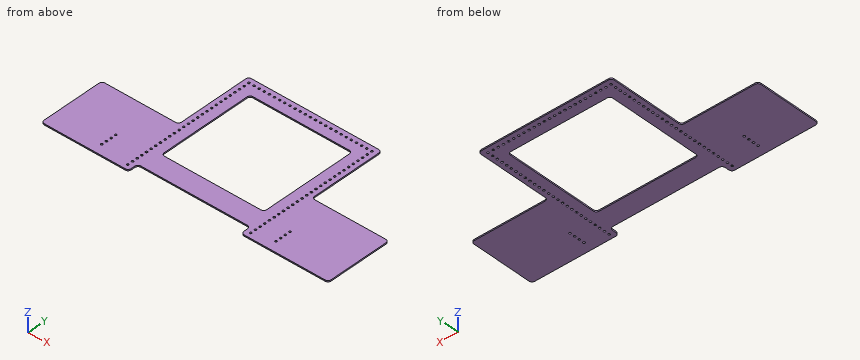
```python
from build123d import *

# Parameters (mm, degrees)
SKETCH1_R           = 2.54
SKETCH1_W           = 254
SKETCH1_H           = 241.3
BOSS_EXTRUDE1_DEPTH = 3.175
FILLET1_R           = 7.62


with BuildPart() as part:
    # Sketch1 → Boss-Extrude1 (new body)
    with BuildSketch(Plane.XY):
        Polygon((392.015739824, -380.530659381), (607.915739824, -380.530659381), (607.915739824, -215.553323478), (417.415739824, -215.553323478), (417.415739824, -25.053323478), (87.215739824, -25.053323478), (87.215739824, -215.553323478), (-103.284260176, -215.553323478), (-103.284260176, -380.530659381), (112.615739824, -380.530659381), (112.615739824, -355.253323478), (392.015739824, -355.253323478), align=None)
        with Locations((99.915739824, -37.753323478)):
            Circle(SKETCH1_R, mode=Mode.SUBTRACT)
        with Locations((112.615739824, -37.753323478)):
            Circle(SKETCH1_R, mode=Mode.SUBTRACT)
        with Locations((125.315739824, -37.753323478)):
            Circle(SKETCH1_R, mode=Mode.SUBTRACT)
        with Locations((138.015739824, -37.753323478)):
            Circle(SKETCH1_R, mode=Mode.SUBTRACT)
        with Locations((150.715739824, -37.753323478)):
            Circle(SKETCH1_R, mode=Mode.SUBTRACT)
        with Locations((163.415739824, -37.753323478)):
            Circle(SKETCH1_R, mode=Mode.SUBTRACT)
        with Locations((176.115739824, -37.753323478)):
            Circle(SKETCH1_R, mode=Mode.SUBTRACT)
        with Locations((188.815739824, -37.753323478)):
            Circle(SKETCH1_R, mode=Mode.SUBTRACT)
        with Locations((201.515739824, -37.753323478)):
            Circle(SKETCH1_R, mode=Mode.SUBTRACT)
        with Locations((214.215739824, -37.753323478)):
            Circle(SKETCH1_R, mode=Mode.SUBTRACT)
        with Locations((226.915739824, -37.753323478)):
            Circle(SKETCH1_R, mode=Mode.SUBTRACT)
        with Locations((239.615739824, -37.753323478)):
            Circle(SKETCH1_R, mode=Mode.SUBTRACT)
        with Locations((252.315739824, -37.753323478)):
            Circle(SKETCH1_R, mode=Mode.SUBTRACT)
        with Locations((265.015739824, -37.753323478)):
            Circle(SKETCH1_R, mode=Mode.SUBTRACT)
        with Locations((277.715739824, -37.753323478)):
            Circle(SKETCH1_R, mode=Mode.SUBTRACT)
        with Locations((290.415739824, -37.753323478)):
            Circle(SKETCH1_R, mode=Mode.SUBTRACT)
        with Locations((303.115739824, -37.753323478)):
            Circle(SKETCH1_R, mode=Mode.SUBTRACT)
        with Locations((315.815739824, -37.753323478)):
            Circle(SKETCH1_R, mode=Mode.SUBTRACT)
        with Locations((328.515739824, -37.753323478)):
            Circle(SKETCH1_R, mode=Mode.SUBTRACT)
        with Locations((341.215739824, -37.753323478)):
            Circle(SKETCH1_R, mode=Mode.SUBTRACT)
        with Locations((353.915739824, -37.753323478)):
            Circle(SKETCH1_R, mode=Mode.SUBTRACT)
        with Locations((366.615739824, -37.753323478)):
            Circle(SKETCH1_R, mode=Mode.SUBTRACT)
        with Locations((379.315739824, -37.753323478)):
            Circle(SKETCH1_R, mode=Mode.SUBTRACT)
        with Locations((392.015739824, -37.753323478)):
            Circle(SKETCH1_R, mode=Mode.SUBTRACT)
        with Locations((404.715739824, -37.753323478)):
            Circle(SKETCH1_R, mode=Mode.SUBTRACT)
        with Locations((99.915739824, -50.453323478)):
            Circle(SKETCH1_R, mode=Mode.SUBTRACT)
        with Locations((99.915739824, -63.153323478)):
            Circle(SKETCH1_R, mode=Mode.SUBTRACT)
        with Locations((99.915739824, -75.853323478)):
            Circle(SKETCH1_R, mode=Mode.SUBTRACT)
        with Locations((99.915739824, -88.553323478)):
            Circle(SKETCH1_R, mode=Mode.SUBTRACT)
        with Locations((99.915739824, -101.253323478)):
            Circle(SKETCH1_R, mode=Mode.SUBTRACT)
        with Locations((99.915739824, -113.953323478)):
            Circle(SKETCH1_R, mode=Mode.SUBTRACT)
        with Locations((99.915739824, -126.653323478)):
            Circle(SKETCH1_R, mode=Mode.SUBTRACT)
        with Locations((99.915739824, -139.353323478)):
            Circle(SKETCH1_R, mode=Mode.SUBTRACT)
        with Locations((99.915739824, -152.053323478)):
            Circle(SKETCH1_R, mode=Mode.SUBTRACT)
        with Locations((99.915739824, -164.753323478)):
            Circle(SKETCH1_R, mode=Mode.SUBTRACT)
        with Locations((99.915739824, -177.453323478)):
            Circle(SKETCH1_R, mode=Mode.SUBTRACT)
        with Locations((99.915739824, -190.153323478)):
            Circle(SKETCH1_R, mode=Mode.SUBTRACT)
        with Locations((99.915739824, -202.853323478)):
            Circle(SKETCH1_R, mode=Mode.SUBTRACT)
        with Locations((99.915739824, -215.553323478)):
            Circle(SKETCH1_R, mode=Mode.SUBTRACT)
        with Locations((99.915739824, -228.253323478)):
            Circle(SKETCH1_R, mode=Mode.SUBTRACT)
        with Locations((99.915739824, -240.953323478)):
            Circle(SKETCH1_R, mode=Mode.SUBTRACT)
        with Locations((99.915739824, -253.653323478)):
            Circle(SKETCH1_R, mode=Mode.SUBTRACT)
        with Locations((99.915739824, -266.353323478)):
            Circle(SKETCH1_R, mode=Mode.SUBTRACT)
        with Locations((99.915739824, -279.053323478)):
            Circle(SKETCH1_R, mode=Mode.SUBTRACT)
        with Locations((99.915739824, -291.753323478)):
            Circle(SKETCH1_R, mode=Mode.SUBTRACT)
        with Locations((99.915739824, -304.453323478)):
            Circle(SKETCH1_R, mode=Mode.SUBTRACT)
        with Locations((99.915739824, -317.153323478)):
            Circle(SKETCH1_R, mode=Mode.SUBTRACT)
        with Locations((99.915739824, -329.853323478)):
            Circle(SKETCH1_R, mode=Mode.SUBTRACT)
        with Locations((99.915739824, -342.553323478)):
            Circle(SKETCH1_R, mode=Mode.SUBTRACT)
        with Locations((99.915739824, -355.253323478)):
            Circle(SKETCH1_R, mode=Mode.SUBTRACT)
        with Locations((99.915739824, -367.953323478)):
            Circle(SKETCH1_R, mode=Mode.SUBTRACT)
        with Locations((404.715739824, -50.453323478)):
            Circle(SKETCH1_R, mode=Mode.SUBTRACT)
        with Locations((404.715739824, -63.153323478)):
            Circle(SKETCH1_R, mode=Mode.SUBTRACT)
        with Locations((404.715739824, -75.853323478)):
            Circle(SKETCH1_R, mode=Mode.SUBTRACT)
        with Locations((404.715739824, -88.553323478)):
            Circle(SKETCH1_R, mode=Mode.SUBTRACT)
        with Locations((404.715739824, -101.253323478)):
            Circle(SKETCH1_R, mode=Mode.SUBTRACT)
        with Locations((404.715739824, -113.953323478)):
            Circle(SKETCH1_R, mode=Mode.SUBTRACT)
        with Locations((404.715739824, -126.653323478)):
            Circle(SKETCH1_R, mode=Mode.SUBTRACT)
        with Locations((404.715739824, -139.353323478)):
            Circle(SKETCH1_R, mode=Mode.SUBTRACT)
        with Locations((404.715739824, -152.053323478)):
            Circle(SKETCH1_R, mode=Mode.SUBTRACT)
        with Locations((404.715739824, -164.753323478)):
            Circle(SKETCH1_R, mode=Mode.SUBTRACT)
        with Locations((404.715739824, -177.453323478)):
            Circle(SKETCH1_R, mode=Mode.SUBTRACT)
        with Locations((404.715739824, -190.153323478)):
            Circle(SKETCH1_R, mode=Mode.SUBTRACT)
        with Locations((404.715739824, -202.853323478)):
            Circle(SKETCH1_R, mode=Mode.SUBTRACT)
        with Locations((404.715739824, -215.553323478)):
            Circle(SKETCH1_R, mode=Mode.SUBTRACT)
        with Locations((404.715739824, -228.253323478)):
            Circle(SKETCH1_R, mode=Mode.SUBTRACT)
        with Locations((404.715739824, -240.953323478)):
            Circle(SKETCH1_R, mode=Mode.SUBTRACT)
        with Locations((404.715739824, -253.653323478)):
            Circle(SKETCH1_R, mode=Mode.SUBTRACT)
        with Locations((404.715739824, -266.353323478)):
            Circle(SKETCH1_R, mode=Mode.SUBTRACT)
        with Locations((404.715739824, -279.053323478)):
            Circle(SKETCH1_R, mode=Mode.SUBTRACT)
        with Locations((404.715739824, -291.753323478)):
            Circle(SKETCH1_R, mode=Mode.SUBTRACT)
        with Locations((404.715739824, -304.453323478)):
            Circle(SKETCH1_R, mode=Mode.SUBTRACT)
        with Locations((404.715739824, -317.153323478)):
            Circle(SKETCH1_R, mode=Mode.SUBTRACT)
        with Locations((404.715739824, -329.853323478)):
            Circle(SKETCH1_R, mode=Mode.SUBTRACT)
        with Locations((404.715739824, -342.553323478)):
            Circle(SKETCH1_R, mode=Mode.SUBTRACT)
        with Locations((404.715739824, -355.253323478)):
            Circle(SKETCH1_R, mode=Mode.SUBTRACT)
        with Locations((404.715739824, -367.953323478)):
            Circle(SKETCH1_R, mode=Mode.SUBTRACT)
        with Locations((23.715739824, -317.153323478)):
            Circle(SKETCH1_R, mode=Mode.SUBTRACT)
        with Locations((455.515739824, -317.153323478)):
            Circle(SKETCH1_R, mode=Mode.SUBTRACT)
        with Locations((455.515739824, -329.853323478)):
            Circle(SKETCH1_R, mode=Mode.SUBTRACT)
        with Locations((455.515739824, -342.553323478)):
            Circle(SKETCH1_R, mode=Mode.SUBTRACT)
        with Locations((455.515739824, -355.253323478)):
            Circle(SKETCH1_R, mode=Mode.SUBTRACT)
        with Locations((23.715739824, -329.853323478)):
            Circle(SKETCH1_R, mode=Mode.SUBTRACT)
        with Locations((23.715739824, -342.553323478)):
            Circle(SKETCH1_R, mode=Mode.SUBTRACT)
        with Locations((23.715739824, -355.253323478)):
            Circle(SKETCH1_R, mode=Mode.SUBTRACT)
        with Locations((252.315739824, -183.803323478)):
            Rectangle(SKETCH1_W, SKETCH1_H, mode=Mode.SUBTRACT)
    extrude(amount=BOSS_EXTRUDE1_DEPTH)

    # Fillet1
    fillet1_edges = [part.edges().sort_by_distance(p)[0] for p in [
        (607.915739824, -380.530659381, 1.5875),
        (392.015739824, -380.530659381, 1.5875),
        (392.015739824, -355.253323478, 1.5875),
        (112.615739824, -355.253323478, 1.5875),
        (112.615739824, -380.530659381, 1.5875),
        (-103.284260176, -380.530659381, 1.5875),
        (-103.284260176, -215.553323478, 1.5875),
        (87.215739824, -215.553323478, 1.5875),
        (87.215739824, -25.053323478, 1.5875),
        (417.415739824, -25.053323478, 1.5875),
        (417.415739824, -215.553323478, 1.5875),
        (607.915739824, -215.553323478, 1.5875),
        (125.315739824, -63.153323478, 1.5875),
        (125.315739824, -304.453323478, 1.5875),
        (379.315739824, -304.453323478, 1.5875),
        (379.315739824, -63.153323478, 1.5875),
    ]]
    fillet(fillet1_edges, radius=FILLET1_R)


solid = part.part
```
Here's how the part is built. I have some questions about the finished solid (model axes, mm). Coordinates: 2 decimals unless noted, no trailing zeros. Order: outer loops, then holes, each group sorted by start corner. A loop starts at its lowest first (then second) coordinate and runs counter-clockwise, first axis right, second up.
Item 1: I'm going to push flat-ended pins straight in: pin 1 Ø1 at (y, z) = (-169, 0.5) entering from -X; pin 2 Ø3 at (x, y) = (404.72, -63.15) entering from -Z; pin 3 Ø1 at (x, z) = (281, 0.5) entering from -Y. Where does each tip first touch, or does it pass through?
Response values:
pin 1: stops at x = 87.22
pin 2: passes through
pin 3: stops at y = -355.25
Item 2: I need wall thicknesses on probe 1 along Y at (x, z) = (227, 2.05); probe 2 along X at (y, z) = (-133, 1.75); probe 3 along Y at (x, z) = (257.5, 1.8). Which ranges of each line are inside material? Lowest first, please.
Response values:
probe 1: y = -355.25 to -304.45, -63.15 to -40.29, -35.21 to -25.05
probe 2: x = 87.22 to 125.32, 379.32 to 417.42
probe 3: y = -355.25 to -304.45, -63.15 to -25.05
Item 3: If we section it at B-B, the plane z = 2.6: Give the number of separate pieces and of enclosed holes in the cut face, then the cut area to 3 significant figures.
Response values:
separate pieces: 1
enclosed holes: 86
area: 110,000 mm2
Item 4: If we section it at A-A, the plane x = 562: List the corners of the cut face in (y, z) for me (3 decimals), then the cut area to 3 significant figures.
Response values:
outline: (-380.531, 0) - (-215.553, 0) - (-215.553, 3.175) - (-380.531, 3.175) - close
area: 524 mm2
